from build123d import *

# Parameters (mm, degrees)
F0_R      = 3.475
F1_DEPTH  = 3.85
F2_R      = 2.425
F3_DEPTH  = 2
F5_DEPTH  = 1
F6_R      = 2.325
F7_DEPTH  = 1
F8_R      = 1.275
F9_DEPTH  = 2.851
F10_R     = 0.5
F11_DEPTH = 3.851


with BuildPart() as f1:
    # F0 (on Top) → F1 (new body)
    with BuildSketch(Plane.XY):
        Circle(F0_R)
    extrude(amount=F1_DEPTH)

    # F2 (on face) → F3 (cut)
    with BuildSketch(Plane(origin=(0, 0, 0), x_dir=(1, 0, 0), z_dir=(0, 0, -1))):
        Circle(F2_R)
    extrude(amount=-F3_DEPTH, mode=Mode.SUBTRACT)

    # F4 (on face) → F5 (join)
    with BuildSketch(Plane.XY.offset(3.85)):
        with BuildLine():
            Line((14.22, 2), (0, 3.475))
            ThreePointArc((0, 3.475), (-3.475, 0), (0, -3.475))
            Line((0, -3.475), (14.22, -2))
            ThreePointArc((14.22, -2), (16.023276, 0), (14.22, 2))
        make_face()
    extrude(amount=-F5_DEPTH)

    # F6 (on face) → F7 (cut)
    with BuildSketch(Plane.XY.offset(3.85)):
        Circle(F6_R)
    extrude(amount=-F7_DEPTH, mode=Mode.SUBTRACT)

    # F8 (on face) → F9 (cut, through all)
    with BuildSketch(Plane.XY.offset(2.85)):
        Circle(F8_R)
    extrude(amount=-F9_DEPTH, mode=Mode.SUBTRACT)

    # F10 (on face) → F11 (cut, through all)
    with BuildSketch(Plane.XY.offset(3.85)):
        with Locations((14.012546, 0)):
            Circle(F10_R)
        with Locations((12.042546, 0)):
            Circle(F10_R)
        with Locations((10.072546, 0)):
            Circle(F10_R)
        with Locations((8.102546, 0)):
            Circle(F10_R)
        with Locations((6.132546, 0)):
            Circle(F10_R)
        with Locations((4.162546, 0)):
            Circle(F10_R)
    extrude(amount=-F11_DEPTH, mode=Mode.SUBTRACT)


solid = f1.part
Work out the finished part from the listing and answer in its coordinate system (mm). A direction names the side the tool comes from. Give positions to 0.01 mm unless a question says otherwise; leave off trailing zeros. Order: outer loops, then holes, each group sorted by start corner. A loop starts at its lowest first (then second) coordinate and runs counter-clockwise, first axis right, second up. Notation, with made-up numbers: (-17, 0.5) -> (16, 0.5) arc R27 cw to (16, 31.5) -> close; hole circle Ø8 at (79.25, -22.5). An arc over 180 degrees is marked (long way). Answer as a JSON object with one key per item and string values. Group by question number.
1. The mould has two halves that part along Y. Classify faces 1 (the flat face through (7.56, 2.69, 3.36)), 2 (the cylindrical face through (-3.47, 0.15, 1.9)), 3 (the cylindrical face through (11.543, 0.022, 3.357)): released by +Y, released by -Y, zero draft, split by the parting line, or undercut.
2. Consider line 1 along Z through (x, y) = (12, 1.25); line 2 along Y through (x, z) = (-2, 1.6); line 3 along Z through (x, y) = (1.25, -1.25). Determine where each line is inside the solid, lowest interval first. Write a range as [from, to].
3. Section D-D on y = -1.75 is taken. Determine the outline of the cut face in (x, z).
4. Section B-B on y = 0 is taken. Count the separate pieces of the cut face and the enclosed holes in it, plus the area to 3 significant figures.
5. A tool of negligible diameter and unlimited length cuts with its end or side. For faces 4 (the cylindrical face through (1.25, 1.96, 3.36)), 5 (the cylindrical face through (4.624, -0.192, 3.357)), 6 (the flat face through (1.04, 1.04, 2)), from which of +Z, -Z, +X, -X, +Y, -Y can it reach the whole face along a straight path? Write none if from no direction.
6. Section A-A on x = 0 is taken. Determine the outline of the cut face in (y, z) (3 decimals), plus the area to 3 significant figures.
7. Section C-C on z = 2.5 is taken. Determine the outline of the cut face in (x, y) (3 decimals).
8. Flat-ended cylindrical pins translate along their axes: pin 1 Ø4 at (x, y) = (0, 0) entering from -Z; pin 2 Ø1.4 at (x, y) = (1, 0.5) entering from +Z; pin 3 Ø2 at (x, y) = (8.5, -0.5) entering from -Z. Find the tip coordinate at first contact, or state that the pin passes through.
Result sheet:
{
 "1": {"face 1": "released by +Y", "face 2": "split by the parting line", "face 3": "undercut"},
 "2": {"line 1": "z = [2.85, 3.85]", "line 2": "y = [-2.84, -1.37], [1.37, 2.84]", "line 3": "z = [2, 2.85]"},
 "3": {"outline": "(-3, 0) -> (-1.68, 0) -> (-1.68, 2) -> (1.68, 2) -> (1.68, 0) -> (3, 0) -> (3, 2.85) -> (15, 2.85) -> (15, 3.85) -> (1.53, 3.85) -> (1.53, 2.85) -> (-1.53, 2.85) -> (-1.53, 3.85) -> (-3, 3.85) -> close"},
 "4": {"separate pieces": "8", "enclosed holes": "0", "area": "16.8 mm^2"},
 "5": {"face 4": "+Z", "face 5": "+Z, -Z", "face 6": "-Z"},
 "6": {"outline": "(-3.475, 0) -> (-2.425, 0) -> (-2.425, 2) -> (-1.275, 2) -> (-1.275, 2.85) -> (-2.325, 2.85) -> (-2.325, 3.85) -> (-3.475, 3.85) -> close; (1.275, 2) -> (2.425, 2) -> (2.425, 0) -> (3.475, 0) -> (3.475, 3.85) -> (2.325, 3.85) -> (2.325, 2.85) -> (1.275, 2.85) -> close", "area": "10.2 mm^2"},
 "7": {"outline": "circle Ø6.95 at (0, 0); hole circle Ø2.55 at (0, 0)"},
 "8": {"pin 1": "stops at z = 2", "pin 2": "stops at z = 2.85", "pin 3": "stops at z = 2.85"}
}
